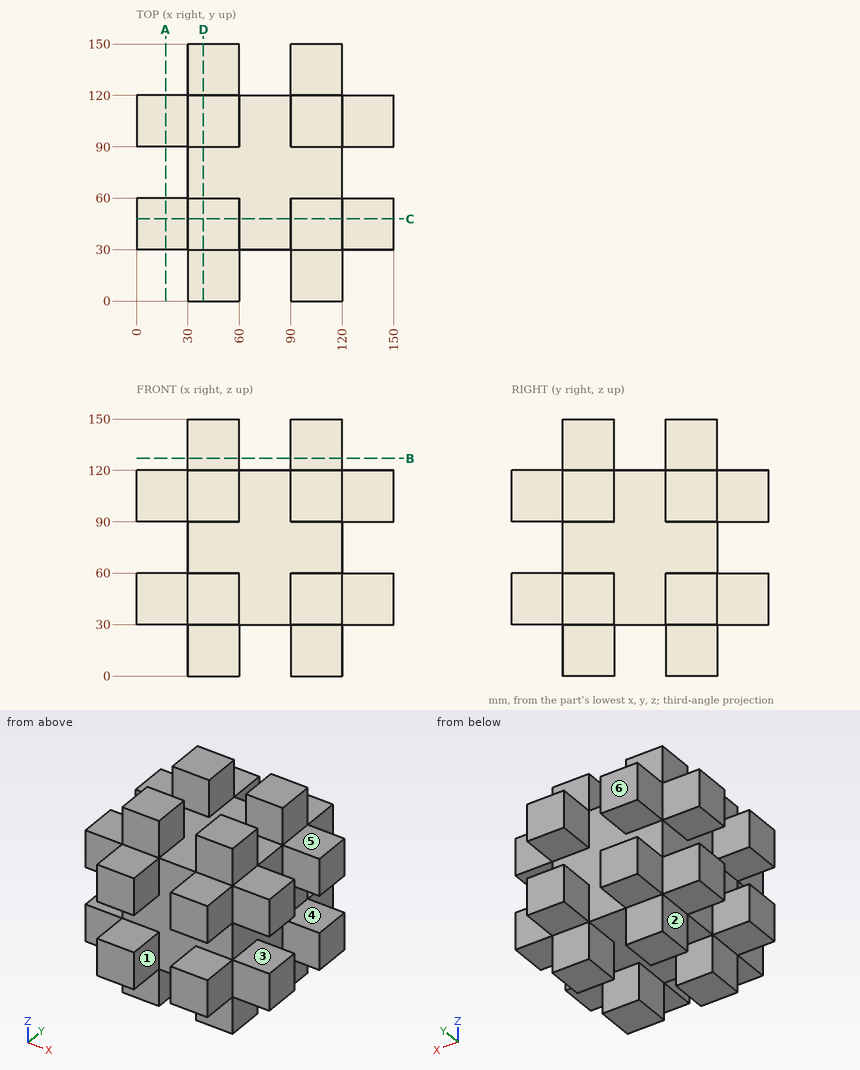
The drawing under review shows one solid part. Ordinate dimensions are in mm from its lowest x, y, z. A direction names the side the tool comes from. Round coordinates to 2 decimals unless told otherwise and drop trailing zeros. Order: outer loops, then holes, each group sorted by start corner. A loop starts at its lowest first (then second) coordinate and runs counter-clockwise, first axis right, second up. Notation, with made-up numbers: (85.5, -17.75) -> (109.5, -17.75) arc R37 cw to (109.5, 20.25) -> close; hole circle Ø9 at (24.25, 25.5). An arc over 180 degrees is marked (long way). Use a Markdown table: item, result.
Item 1: Take a section at C-C (y = 48). State the section outline as (x, z) points, plus the area to 3 significant figures.
Resolved:
| item | result |
|---|---|
| outline | (0, 30) -> (30, 30) -> (30, 0) -> (60, 0) -> (60, 30) -> (90, 30) -> (90, 0) -> (120, 0) -> (120, 30) -> (150, 30) -> (150, 60) -> (120, 60) -> (120, 90) -> (150, 90) -> (150, 120) -> (120, 120) -> (120, 150) -> (90, 150) -> (90, 120) -> (60, 120) -> (60, 150) -> (30, 150) -> (30, 120) -> (0, 120) -> (0, 90) -> (30, 90) -> (30, 60) -> (0, 60) -> close |
| area | 15,300 mm² |
Item 2: Draft analysis for pull direction Z (two halves, no side actions). For the marked faces 4, 5 and 6, state which applies: +Z half, -Z half, draft (parallel to the pull), parting line (faces both ways), or undercut.
Resolved:
| item | result |
|---|---|
| face 4 | undercut |
| face 5 | +Z half |
| face 6 | draft |
Item 3: For pin 1 (15 mm diameter, centred on x = 108.5, y = 133.5, fed in from -Z); pin 2 (5 mm diameter, centred on x = 79.5, z = 61.5, fed in from +Y); pin 3 (9 mm diameter, centred on y = 109.5, z = 16, fed in from +X); pin 4 (1.5 mm diameter, centred on y = 48.5, z = 41.5, fed in from -X), all flat-tipped, find the tip position at first contact; note any pin that passes through.
Resolved:
| item | result |
|---|---|
| pin 1 | stops at z = 30 |
| pin 2 | stops at y = 120 |
| pin 3 | stops at x = 120 |
| pin 4 | stops at x = 0 |
Item 4: Machinability: for the marked faces 1, 2 and 3, which of the approach directions +Z, -Z, +X, -X, +Y, -Y give a long, thin tool a straight path to every point of the face, cutting with its end or side? Answer none if there is none.
Resolved:
| item | result |
|---|---|
| face 1 | +Z, -Z, -Y |
| face 2 | -Z, -X, +Y, -Y |
| face 3 | +X, +Y, -Y |
Item 5: Take a section at A-A (x = 17). State the section outline as (y, z) points.
Resolved:
| item | result |
|---|---|
| outline | (30, 30) -> (60, 30) -> (60, 60) -> (30, 60) -> close; (30, 90) -> (60, 90) -> (60, 120) -> (30, 120) -> close; (90, 30) -> (120, 30) -> (120, 60) -> (90, 60) -> close; (90, 90) -> (120, 90) -> (120, 120) -> (90, 120) -> close |
Item 6: For line 1 along Z through (x, y) = (24, 36), list the stretches that pass through material, from the lowest coordinate up. Write a range as [from, to].
Resolved:
| item | result |
|---|---|
| line 1 | z = [30, 60], [90, 120] |
